Check sheet for the modelled part. Datum: model origin and axes. Units: mm. Face numbers are marked on the shaded views. A direction names the side the tool comes from. Coordinates: 2 decimals unless noted, no trailing zeros. Loops run counter-clockwise (first coordinate to the right, second up) from the corner with the lowest first, then second, coordinate; pieces in that order, holes last.
```python
from build123d import *

# Parameters (mm, degrees)
F1_DEPTH = 80
F3_D     = 5.5
F4_SIZE  = 5
F5_R     = 1


with BuildPart() as f1:
    # F0 (on Front) → F1 (new body)
    with BuildSketch(Plane.XZ):
        Polygon((0, 20), (0, 0), (29, 0), (29, -79), (30, -79), (30, 1), (1, 1), (1, 20), align=None)
    extrude(amount=F1_DEPTH)

    # F3 (through all)
    with Locations(Plane.YZ.offset(1)):
        with Locations((-73.2, 13.2), (-6.8, 13.2)):
            Hole(F3_D / 2)

    # F4
    f4_edges = [f1.edges().sort_by_distance(p)[0] for p in [
        (0.5, -80, 20),
        (0.5, 0, 20),
        (29.5, 0, -79),
        (29.5, -80, -79),
    ]]
    chamfer(f4_edges, length=F4_SIZE)

    # F5
    f5_edges = [f1.edges().sort_by_distance(p)[0] for p in [
        (30, -40, 1),
        (0, -40, 0),
    ]]
    fillet(f5_edges, radius=F5_R)


solid = f1.part
```
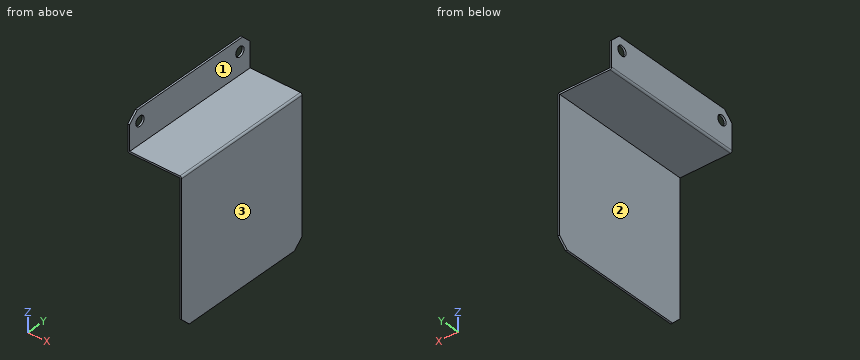
1) Section check C-C on y = -40. Enter the section's corners in (x, z).
Answer sheet:
outline: (0, 1) arc R1 ccw to (1, 0) - (29, 0) - (29, -79) - (30, -79) - (30, 0) arc R1 ccw to (29, 1) - (1, 1) - (1, 20) - (0, 20) - close
2) Section check B-B on y = -73.2. Enter the section's corners in (x, z).
Answer sheet:
outline: (0, 1) arc R1 ccw to (1, 0) - (29, 0) - (29, -79) - (30, -79) - (30, 0) arc R1 ccw to (29, 1) - (1, 1) - (1, 10.45) - (0, 10.45) - close; (0, 15.95) - (1, 15.95) - (1, 20) - (0, 20) - close
3) Section check D-D on x = 21.5. Enter the section's corners in (y, z), plus the area to 3 significant figures.
Answer sheet:
outline: (-80, 0) - (0, 0) - (0, 1) - (-80, 1) - close
area: 80.0 mm2
4) Scan lines: line 1 (Z direction, x = 0.85, y = -73.2); line 2 (X direction, y = -21.5, z = -1); line 3 (Z direction, x = 7.25, y = -41). Record each from-to range of solid material in increasing order.
Answer sheet:
line 1: z = 0.01 to 10.45, 15.95 to 20
line 2: x = 29 to 30
line 3: z = 0 to 1
5) Depth check by flat-ended pin: pin 1 (4 mm diameter, centred on y = -62, z = -66.5, fed in from -X); pin 2 (10 mm diameter, centred on x = 22.5, y = -17.5, fed in from +Z); pin 3 (9.5 mm diameter, centred on y = -26, z = 10.5, fed in from +X). Enter the tip coordinate at first touch or a pass-through.
Answer sheet:
pin 1: stops at x = 29
pin 2: stops at z = 1
pin 3: stops at x = 1
6) Set-up check for the marked faces 1, 2 and 3: record each of +Z, -Z, +X, -X, +Y, -Y from which the full face is reachable in a straight line by a thin tool's end or side.
Answer sheet:
face 1: +Z, +X, +Y, -Y
face 2: -Z, -X, +Y, -Y
face 3: +Z, -Z, +X, +Y, -Y
7) Section check A-A on z = 13.2. Enter the section's corners in (x, y).
Answer sheet:
outline: (0, -80) - (1, -80) - (1, -75.95) - (0, -75.95) - close; (0, -70.45) - (1, -70.45) - (1, -9.55) - (0, -9.55) - close; (0, -4.05) - (1, -4.05) - (1, 0) - (0, 0) - close
